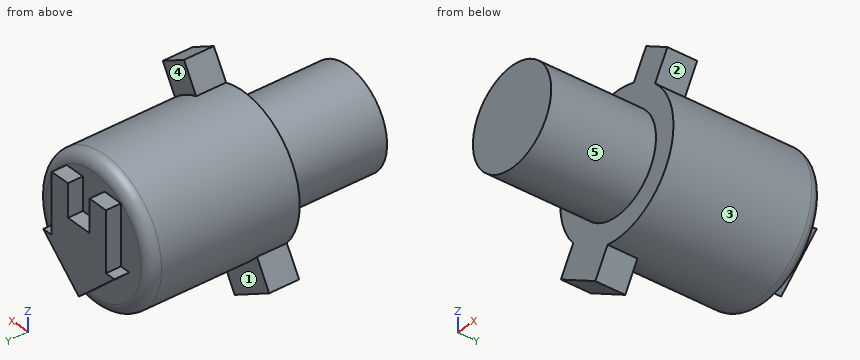
from build123d import *

# Parameters (mm, degrees)
SKETCH1_R           = 3.25
BOSS_EXTRUDE1_DEPTH = 7.018
SKETCH6_R           = 4.7
BOSS_EXTRUDE2_DEPTH = 10
BOSS_EXTRUDE3_DEPTH = 1
FILLET1_R           = 0.75
BOSS_EXTRUDE4_DEPTH = 2


with BuildPart() as part:
    # Sketch1 → Boss-Extrude1 (new body)
    with BuildSketch(Plane(origin=(0, 0, 0), x_dir=(1, 0, 0), z_dir=(0, 1, 0))):
        Circle(SKETCH1_R)
    extrude(amount=BOSS_EXTRUDE1_DEPTH)

    # Sketch6 → Boss-Extrude2 (add)
    with BuildSketch(Plane(origin=(0, 7.018, 0), x_dir=(1, 0, 0), z_dir=(0, 1, 0))):
        Circle(SKETCH6_R)
    extrude(amount=BOSS_EXTRUDE2_DEPTH)

    # Sketch12 → Boss-Extrude3 (add)
    with BuildSketch(Plane(origin=(0, 17.018, 0), x_dir=(1, 0, 0), z_dir=(0, 1, 0))):
        Polygon((0, 3.542487974), (-2.95, 0.842487974), (-2.25, 0.842487974), (-2.25, -3.157512026), (-0.9, -3.172366953), (-0.9, -0.972366953), (0.9, -0.972366953), (0.9, -3.172366953), (2.25, -3.157512026), (2.25, 0.842487974), (2.95, 0.842487974), align=None)
    extrude(amount=BOSS_EXTRUDE3_DEPTH)

    # Fillet1
    fillet1_edges = [part.edges().sort_by_distance(p)[0] for p in [
        (-4.7, 17.018, 0),
    ]]
    fillet(fillet1_edges, radius=FILLET1_R)

    # Sketch13 → Boss-Extrude4 (add)
    with BuildSketch(Plane.XZ.offset(-7.018)):
        with BuildLine():
            Line((-0.770430625, -4.636424986), (-1.786430625, -6.396188607))
            Line((-1.786430625, -6.396188607), (-4.646046508, -4.745188607))
            Line((-4.646046508, -4.745188607), (-3.630046508, -2.985424986))
            ThreePointArc((-3.630046508, -2.985424986), (-2.35, -4.070319398), (-0.770430625, -4.636424986))
        make_face()
        with BuildLine():
            Line((3.174317689, 3.466079516), (4.190317689, 5.225843137))
            Line((4.190317689, 5.225843137), (2.430554068, 6.241843137))
            Line((2.430554068, 6.241843137), (1.414554068, 4.482079516))
            ThreePointArc((1.414554068, 4.482079516), (2.35, 4.070319398), (3.174317689, 3.466079516))
        make_face()
    extrude(amount=-BOSS_EXTRUDE4_DEPTH)


solid = part.part
Part model, mm, in its own coordinate system. Face numbers are marked on the shaded views. A direction names the side the tool comes from. Coordinates: 2 decimals unless noted, no trailing zeros. Loops run counter-clockwise (first coordinate to the right, second up) from the corner with the lowest first, then second, coordinate; pieces in that order, holes last. Notation, with made-up numbers: (80.5, 1.5) - (103.5, 1.5) arc R20 ccw to (103.5, 13.5) - close; hole circle Ø8 at (-16.5, 4.25). An arc over 180 degrees is marked (long way). Write each question's results on one line, items separated by ' | '. Start each with the question number.
Q1. Slice it at D-D on y = 14. Give the cut face in (x, z).
Q2. Which spindle directions (+Z, -Z, +X, -X, +Y, -Y) get a long thin tool onto all of the face, cutting with end or side? Do the marked faces 1, 2, 3, 4 and 5. Say none if no direction does.
Q3. Probe line 1 along Y through (x, z) = (-4, -0.5); line 2 along Y through (x, z) = (-3.5, -3.5); line 3 along Z through (x, y) = (1.75, 1.5). List the from-to ranges inside material, lowest first.
Q4. Slice it at A-A on z = 0. Give the cut face in (x, y), and give its area (3 significant figures).
Q5. Drop flat-ended pins along their axis: pin 1 Ø0.8 at (x, z) = (2.5, 5) entering from +Y; pin 2 Ø1 at (x, z) = (0, -4) entering from +Y; pin 3 Ø2.5 at (x, z) = (-2.5, -4.5) entering from +Y; pin 4 Ø0.8 at (y, z) = (17.5, 1.5) entering from +X. Give the stop position or say it passes through.
Q6. Slice it at B-B on y = 8. Give the cut face in (x, z), and give its area (3 significant figures).
Q7. Slice it at C-C on y = 2. Give the cut face in (x, z).
Answer:
1) outline: circle Ø9.4 at (0, 0)
2) face 1: -Z, -X, +Y | face 2: +X, +Y, -Y | face 3: +Y | face 4: +Z, +X, +Y | face 5: -Y
3) line 1: y = 7.02 to 17.01 | line 2: y = 7.02 to 9.02 | line 3: z = -2.74 to 2.74
4) outline: (-4.7, 7.02) - (-3.25, 7.02) - (-3.25, 0) - (3.25, 0) - (3.25, 7.02) - (4.7, 7.02) - (4.7, 16.27) arc R0.75 ccw to (3.95, 17.02) - (2.25, 17.02) - (2.25, 18.02) - (-2.25, 18.02) - (-2.25, 17.02) - (-3.95, 17.02) arc R0.75 ccw to (-4.7, 16.27) - close | area: 144 mm2
5) pin 1: stops at y = 9.02 | pin 2: stops at y = 18.02 | pin 3: stops at y = 17.02 | pin 4: stops at x = 2.25
6) outline: (-4.65, -4.75) - (-1.79, -6.4) - (-0.77, -4.64) arc R4.7 ccw to (3.17, 3.47) - (4.19, 5.23) - (2.43, 6.24) - (1.41, 4.48) arc R4.7 ccw to (-3.63, -2.99) - close | area: 79.4 mm2
7) outline: circle Ø6.5 at (0, 0)
